from build123d import *

# Parameters (mm, degrees)
SKETCH1_W               = 30.2
SKETCH1_H               = 30.2
BOSS_EXTRUDE1_DEPTH     = 5
SKETCH2_R               = 13.5
BOSS_EXTRUDE2_DEPTH     = 1
SKETCH3_R               = 2.5
CUT_EXTRUDE1_DEPTH      = 4.5
SKETCH4_R               = 13.5
SKETCH4_R_2             = 12.5
BOSS_EXTRUDE3_DEPTH     = 3
CUT_EXTRUDE2_DEPTH      = 5
CUT_EXTRUDE2_DEPTH_BACK = 5
SKETCH5_R               = 5
BOSS_EXTRUDE4_DEPTH     = 4.5
SKETCH7_R               = 1
SKETCH7_R_2             = 0.5
CUT_SWEEP1_START        = 4.580551388
CUT_SWEEP1_OUTLINE_R    = 0.5
CUT_SWEEP1_DEPTH        = 18.125062915
SKETCH10_R              = 2.5
CUT_EXTRUDE3_DEPTH      = 3
SKETCH12_W              = 3.2
SKETCH12_H              = 3.2
BOSS_EXTRUDE5_DEPTH     = 21
SKETCH15_R              = 1.1
CUT_EXTRUDE4_DEPTH      = 1


# Read off the part's stored shape, not the designer's step: Cut-Sweep1
with BuildPart() as part:
    # Sketch1 → Boss-Extrude1 (new body)
    with BuildSketch(Plane(origin=(0, 0, 0), x_dir=(1, 0, 0), z_dir=(0, 1, 0))):
        with Locations((7.605614303, 19.014035757)):
            Rectangle(SKETCH1_W, SKETCH1_H)
    extrude(amount=BOSS_EXTRUDE1_DEPTH)

    # Sketch2 → Boss-Extrude2 (add)
    with BuildSketch(Plane(origin=(0, 5, 0), x_dir=(1, 0, 0), z_dir=(0, 1, 0))):
        with Locations(Location((7.605614303, 19.014035757, 0), (0, 0, 270))):
            Circle(SKETCH2_R)
    extrude(amount=BOSS_EXTRUDE2_DEPTH)

    # Sketch3 → Cut-Extrude1 (cut)
    with BuildSketch(Plane(origin=(0, 6, 0), x_dir=(1, 0, 0), z_dir=(0, 1, 0))):
        with Locations(Location((7.605614303, 19.014035757, 0), (0, 0, 270))):
            Circle(SKETCH3_R)
    extrude(amount=-CUT_EXTRUDE1_DEPTH, mode=Mode.SUBTRACT)

    # Sketch4 → Boss-Extrude3 (add)
    with BuildSketch(Plane(origin=(0, 6, 0), x_dir=(1, 0, 0), z_dir=(0, 1, 0))):
        with Locations(Location((7.605614303, 19.014035757, 0), (0, 0, 270))):
            Circle(SKETCH4_R)
        with Locations(Location((7.605614303, 19.014035757, 0), (0, 0, 270))):
            Circle(SKETCH4_R_2, mode=Mode.SUBTRACT)
    extrude(amount=BOSS_EXTRUDE3_DEPTH)

    # Sketch5 → Cut-Extrude2 (cut, two sides: drawn at the far end of the back side and taken through both)
    with BuildSketch(Plane(origin=(0, 6, 0), x_dir=(1, 0, 0), z_dir=(0, 1, 0)).offset(-CUT_EXTRUDE2_DEPTH_BACK)):
        with Locations(Location((-0.394385697, 19.014035757, 0), (0, 0, 147.20617704))):
            Circle(SKETCH5_R)
    extrude(amount=CUT_EXTRUDE2_DEPTH + CUT_EXTRUDE2_DEPTH_BACK, mode=Mode.SUBTRACT)

    # Sketch6 → Boss-Extrude4 (add)
    with BuildSketch(Plane(origin=(0, 1, 0), x_dir=(1, 0, 0), z_dir=(0, 1, 0))):
        with BuildLine():
            ThreePointArc((1.019827865, 19.514035757), (-0.394385697, 20.514035757), (-1.80859926, 19.514035757))
            Line((-1.80859926, 19.514035757), (1.019827865, 19.514035757))
        make_face()
        with BuildLine():
            Line((1.019827865, 18.514035757), (-1.80859926, 18.514035757))
            ThreePointArc((-1.80859926, 18.514035757), (-0.394385697, 17.514035757), (1.019827865, 18.514035757))
        make_face()
    extrude(amount=BOSS_EXTRUDE4_DEPTH)

    # Sweep1: sweep along a path in Sketch8
    with BuildLine(Plane(origin=(0, 5, 0), x_dir=(1, 0, 0), z_dir=(0, 1, 0))) as sweep1_path:
        Line((22.705614303, 19.014035757), (4.605614303, 19.014035757))
    # Sketch7 → Sweep1 (sweep)
    with BuildSketch(Plane(origin=(22.705614303, 0, 0), x_dir=(0, 0, -1), z_dir=(1, 0, 0))):
        with Locations((19.014035757, 5)):
            Circle(SKETCH7_R)
        with Locations((19.014035757, 5)):
            Circle(SKETCH7_R_2, mode=Mode.SUBTRACT)
    sweep(path=sweep1_path.line)

    # Cut-Sweep1 outline → Cut-Sweep1 (cut)
    with BuildSketch(Plane.YZ.offset(CUT_SWEEP1_START)):
        with Locations((5, -19.014035757)):
            Circle(CUT_SWEEP1_OUTLINE_R)
    extrude(amount=CUT_SWEEP1_DEPTH, mode=Mode.SUBTRACT)

    # Sketch10 → Cut-Extrude3 (cut)
    with BuildSketch(Plane(origin=(0, 6, 0), x_dir=(1, 0, 0), z_dir=(0, 1, 0))):
        with Locations(Location((7.605614303, 19.014035757, 0), (0, 0, 270))):
            Circle(SKETCH10_R)
    extrude(amount=-CUT_EXTRUDE3_DEPTH, mode=Mode.SUBTRACT)

    # Sketch12 → Boss-Extrude5 (add)
    with BuildSketch(Plane(origin=(0, 5, 0), x_dir=(1, 0, 0), z_dir=(0, 1, 0))):
        with Locations((-5.894385697, 5.514035757)):
            Rectangle(SKETCH12_W, SKETCH12_H)
        with Locations((21.105614303, 5.514035757)):
            Rectangle(SKETCH12_W, SKETCH12_H)
        with Locations((21.105614303, 32.514035757)):
            Rectangle(SKETCH12_W, SKETCH12_H)
        with Locations((-5.894385697, 32.514035757)):
            Rectangle(SKETCH12_W, SKETCH12_H)
    extrude(amount=BOSS_EXTRUDE5_DEPTH)

    # Sketch15 → Cut-Extrude4 (cut)
    with BuildSketch(Plane(origin=(0, 26, 0), x_dir=(1, 0, 0), z_dir=(0, 1, 0))):
        with Locations(Location((-5.894385697, 5.514035757, 0), (0, 0, 270))):
            Circle(SKETCH15_R)
        with Locations(Location((-5.894385697, 32.514035757, 0), (0, 0, 270))):
            Circle(SKETCH15_R)
        with Locations(Location((21.105614303, 32.514035757, 0), (0, 0, 270))):
            Circle(SKETCH15_R)
        with Locations(Location((21.105614303, 5.514035757, 0), (0, 0, 270))):
            Circle(SKETCH15_R)
    extrude(amount=-CUT_EXTRUDE4_DEPTH, mode=Mode.SUBTRACT)


solid = part.part
Check sheet for the modelled part. Datum: model origin and axes. Units: mm. A direction names the side the tool comes from. Round coordinates to 2 decimals unless told otherwise and drop trailing zeros. Loops run counter-clockwise (first coordinate to the right, second up) from the corner with the lowest first, then second, coordinate; pieces in that order, holes last. Notation, with made-up numbers: (9.25, 44) - (29.25, 44) arc R27 cw to (29.25, 83) - close; hole circle Ø11 at (-14.5, 2). An arc over 180 degrees is marked (long way). Answer as CSV lines item,"result". Start each with the question number.
Item 1: Set-up check for faces 1 (the flat face through (0, 5.5, -20)), 2 (the cylindrical face through (22, 6, -19)), 3 (the cylindrical face through (16.29, 4.89, -19.5)): record each of +Z, -Z, +X, -X, +Y, -Y from which the full face is reachable in a straight line by a thin tool's end or side.
Item 2: Section check B-B (y = 6.75). Record the boundary of the cut face in (x, z), and give its area (3 significant figures).
Item 3: Depth check by flat-ended pin: P1, Ø2, axis at y = 13, z = -8.5, coming from the +X side; P2, Ø1.1, axis at x = 0, z = -20, coming from the +Y side; P3, Ø1, axis at x = 9.5, y = 8.5, coming from the +Z side; P4, Ø8, axis at x = 0, z = -21, coming from the +Y side. Enter the tip coordinate at first touch or a pass-through.
Item 4: Section check D-D (x = 15). Record the boundary of the cut face in (y, z).
Item 5: Section check A-A (y = 19.25). Record the boundary of the cut face in (x, z).
Item 6: Section check C-C (z = -29). Record the boundary of the cut face in (x, y), and give its area (3 significant figures).
Item 7: Release check for a two-part mould opening along Z. For faces 4 (the flat face through (0, 5.5, -18)), 5 (the cylindrical face through (5.39, 3.78, -17.86)), 6 (the flat face through (19.506, 15, -32)), 7 (the flat face through (7, 4, -34.114)) record: +Z half, -Z half, draft (parallel to the pull), parting line (faces both ways), or undercut.
Item 8: Scan lines: line 1 (Y direction, x = 17.5, z = -19); line 2 (X direction, y = 6.25, z = -33); line 3 (Z direction, x = 0, y = 4). Record each from-to range of solid material in increasing order. Write a range as [from, to].
Report:
1,face 1,"+Y"
1,face 2,"+X, +Y"
1,face 3,"+X"
2,outline,"(-7.49, -34.11) - (-4.29, -34.11) - (-4.29, -30.91) - (-7.49, -30.91) - close; (-7.49, -7.11) - (-4.29, -7.11) - (-4.29, -3.91) - (-7.49, -3.91) - close; circle Ø27 at (7.61, -19.01); (19.51, -34.11) - (22.71, -34.11) - (22.71, -30.91) - (19.51, -30.91) - close; (19.51, -7.11) - (22.71, -7.11) - (22.71, -3.91) - (19.51, -3.91) - close; hole (-4.6, -21.72) arc R12.5 ccw (long way) to (-4.6, -16.31) arc R5 ccw to start"
2,area,"121 mm2"
3,P1,"passes through"
3,P2,"stops at y = 5.5"
3,P3,"stops at z = -5.59"
3,P4,"stops at y = 6"
4,outline,"(0, -34.11) - (5, -34.11) - (5, -30.31) - (9, -30.31) - (9, -29.09) - (6, -29.09) - (6, -8.94) - (9, -8.94) - (9, -7.72) - (5, -7.72) - (5, -3.91) - (0, -3.91) - close; hole circle Ø1 at (5, -19.01)"
5,outline,"(-7.49, -34.11) - (-4.29, -34.11) - (-4.29, -30.91) - (-7.49, -30.91) - close; (-7.49, -7.11) - (-4.29, -7.11) - (-4.29, -3.91) - (-7.49, -3.91) - close; (19.51, -34.11) - (22.71, -34.11) - (22.71, -30.91) - (19.51, -30.91) - close; (19.51, -7.11) - (22.71, -7.11) - (22.71, -3.91) - (19.51, -3.91) - close"
6,outline,"(-7.49, 0) - (22.71, 0) - (22.71, 5) - (16.69, 5) - (16.69, 9) - (15.12, 9) - (15.12, 6) - (0.09, 6) - (0.09, 9) - (-1.48, 9) - (-1.48, 5) - (-7.49, 5) - close"
6,area,"179 mm2"
7,face 4,"undercut"
7,face 5,"undercut"
7,face 6,"draft"
7,face 7,"-Z half"
8,line 1,"y = [0, 4.5], [5.5, 6]"
8,line 2,"x = [-7.49, -4.29], [19.51, 22.71]"
8,line 3,"z = [-34.11, -24], [-20.46, -19.51], [-18.51, -17.57], [-14.03, -3.91]"
